Source: CAD feature listing. Evaluate the final solid. Frame: model axes, mm. Face numbers are marked on the shaded views. Round coordinates to 2 decimals unless told otherwise and drop trailing zeros. Loops run counter-clockwise (first coordinate to the right, second up) from the corner with the lowest first, then second, coordinate; pieces in that order, holes last.
Item 1: Pull-direction query (X, two-part tool) for the marked faces 1, 2 and 3; classes: released by +X, released by -X, zero draft, split by the parting line, or undercut.
Item 2: Section query D-D on y = 0.5. Return loops of the section in (x, z), then the cut area to 3 significant figures.
Item 3: Ray query, L1, parallel to Z at x = 0, y = 14; L2, parallel to Y at x = 5.5, z = 9; L3, parallel to X at y = -11.5, z = 2.5. Return the intervals inside material, ascending.
Item 4: Section query C-C on z = 5. Return loops of the section in (x, y), then the cut area to 3 significant figures.
Item 5: First-contact query: P1, Ø10, axis at x = -11, z = 6.5, coming from the -Y side; P2, Ø3, axis at x = 8, y = -10.5, coming from the +Z side; P3, Ø4, axis at y = 4.5, z = 14.5, coming from the -X side; P4, Ø12, axis at x = 3, y = -5.5, coming from the +Z side. Flat tips, straight axial feed; report the tip coordinate or a pass-through.
Item 6: Section query B-B on x = 8.5. Return loops of the section in (y, z), then the cut area to 3 significant figures.
Item 7: Section query A-A on x = 0. Return loops of the section in (y, z), then the cut area to 3 significant figures.
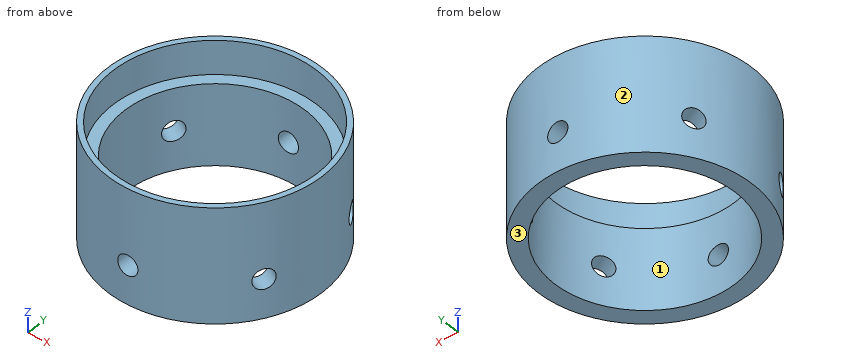
```python
from build123d import *

# Parameters (mm, degrees)
F0_R     = 15.9
F0_R_2   = 13.4
F1_DEPTH = 12
F2_R     = 1.5
F3_DEPTH = 50
F5_COUNT = 3
F7_R     = 15.9
F7_R_2   = 15.1
F8_DEPTH = 5


with BuildPart() as f1:
    # F0 (on Top) → F1 (new body)
    with BuildSketch(Plane.XY):
        Circle(F0_R)
        Circle(F0_R_2, mode=Mode.SUBTRACT)
    extrude(amount=F1_DEPTH)


with BuildPart() as f3:
    # F2 (on Front) → F3 (new body)
    with BuildSketch(Plane.XZ):
        with Locations((0, 5.772834)):
            Circle(F2_R)
    extrude(amount=F3_DEPTH)


with BuildPart() as f3_1:
    # F4: moved
    add(f3.part.moved(Location((0, 25.2, 0))))


with BuildPart() as f5_1:
    # F5: instance of F3
    add(f3_1.part.rotate(Axis((0, 0, 0), (0, 0, -1)), 1 * 360 / F5_COUNT))


with BuildPart() as f5_2:
    # F5: instance of F3
    add(f3_1.part.rotate(Axis((0, 0, 0), (0, 0, -1)), 2 * 360 / F5_COUNT))


with BuildPart() as f1_1:
    add(f1.part)

    # F6: cut F5_1, F3, F5_2
    add(f5_1.part, mode=Mode.SUBTRACT)
    add(f3_1.part, mode=Mode.SUBTRACT)
    add(f5_2.part, mode=Mode.SUBTRACT)

    # F7 (on face) → F8 (join)
    with BuildSketch(Plane.XY.offset(12)):
        Circle(F7_R)
        Circle(F7_R_2, mode=Mode.SUBTRACT)
    extrude(amount=F8_DEPTH)


solid = f1_1.part
```
Data:
1. face 1: undercut
1. face 2: split by the parting line
1. face 3: zero draft
2. outline: (-15.89, 0) - (-13.39, 0) - (-13.39, 12) - (-15.09, 12) - (-15.09, 17) - (-15.89, 17) - close; (13.39, 0) - (15.89, 0) - (15.89, 17) - (15.09, 17) - (15.09, 12) - (13.39, 12) - close
2. area: 68.0 mm2
3. L1: z = 0 to 4.27, 7.27 to 12
3. L2: y = -14.92 to -12.22, 12.22 to 14.92
3. L3: x = -10.98 to -6.88, 6.88 to 10.98
4. outline: (-14.37, -6.81) - (-12.19, -5.56) arc R13.4 cw to (-12.19, 5.56) - (-14.37, 6.81) arc R15.9 ccw to start; (-13.08, -9.04) arc R15.9 ccw to (-1.29, -15.85) - (-1.29, -13.34) arc R13.4 cw to (-10.91, -7.78) - close; (-13.08, 9.04) - (-10.91, 7.78) arc R13.4 cw to (-1.29, 13.34) - (-1.29, 15.85) arc R15.9 ccw to start; (1.29, -15.85) arc R15.9 ccw to (13.08, -9.04) - (10.91, -7.78) arc R13.4 cw to (1.29, -13.34) - close; (1.29, 13.34) arc R13.4 cw to (10.91, 7.78) - (13.08, 9.04) arc R15.9 ccw to (1.29, 15.85) - close; (12.19, -5.56) - (14.37, -6.81) arc R15.9 ccw to (14.37, 6.81) - (12.19, 5.56) arc R13.4 cw to start
4. area: 192 mm2
5. P1: stops at y = -14.72
5. P2: stops at z = 12
5. P3: stops at x = -15.7
5. P4: passes through
6. outline: (-13.44, 0) - (-10.36, 0) - (-10.36, 12) - (-12.48, 12) - (-12.48, 17) - (-13.44, 17) - close; (10.36, 0) - (13.44, 0) - (13.44, 17) - (12.48, 17) - (12.48, 12) - (10.36, 12) - close
6. area: 83.4 mm2
7. outline: (-15.9, 0) - (-13.4, 0) - (-13.4, 4.27) - (-15.9, 4.27) - close; (-15.9, 7.27) - (-13.4, 7.27) - (-13.4, 12) - (-15.1, 12) - (-15.1, 17) - (-15.9, 17) - close; (13.4, 0) - (15.9, 0) - (15.9, 4.27) - (13.4, 4.27) - close; (13.4, 7.27) - (15.9, 7.27) - (15.9, 17) - (15.1, 17) - (15.1, 12) - (13.4, 12) - close
7. area: 53.0 mm2
